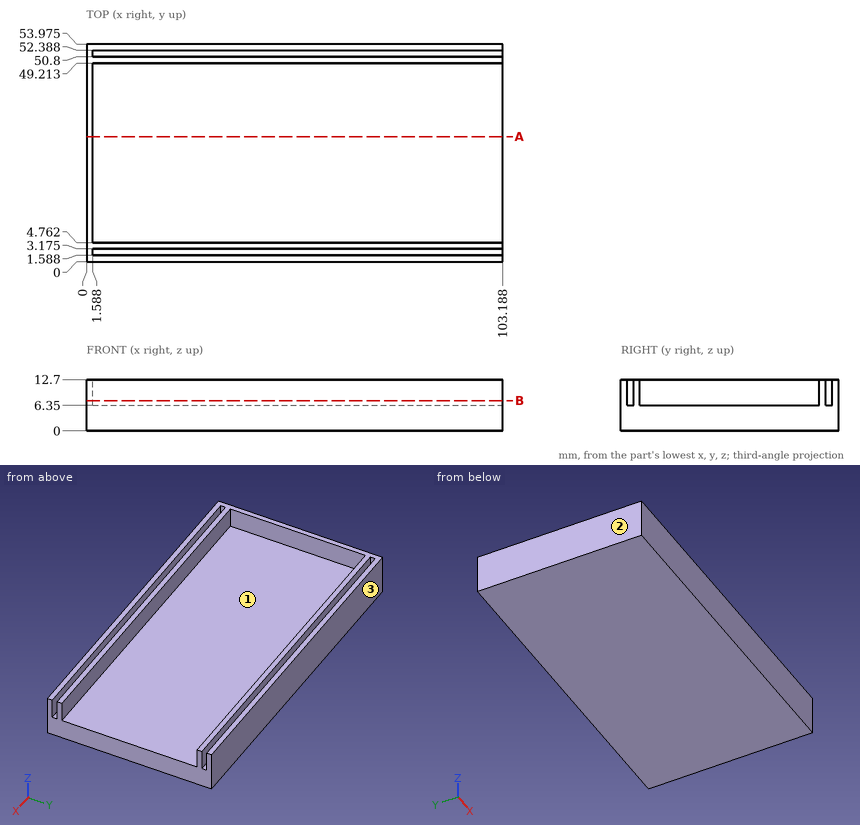
Here's the drawing with two shaded views (mm, measured from the low corner). I have some questions. Round coordinates to 2 decimals unless told otherwise and drop trailing zeros. Order: outer loops, then holes, each group sorted by start corner. A loop starts at its lowest first (then second) coordinate and runs counter-clockwise, first axis right, second up. Notation, with made-up numbers: (58.25, -5) -> (105.25, -5) arc R14 ccw to (105.25, 5) -> close; hole circle Ø7 at (53, -39). An arc over 180 degrees is marked (long way). Use a Markdown table: item, result. Add a question column.
(1) For pin 1 Ø12 at (x, y) = (19.5, 25.5) entering from +Z; pin 2 Ø1.9 at (y, z) = (26.5, 10) entering from +X, each with a flat end and sliding along its axis, tell me the tip position at first contact or that it passes through.
(2) Suppose I cut it at B-B, the plane z = 7.5. Please give me the cut outline in (x, y) (1 decimal).
(3) Suppose I cut it at A-A, the plane y = 31. Please give me the cut outline in (x, z).
(4) If we mould it in two halves opening along Y, with no side actions, what happens to the marked faces 1, 2 and 3? For each: released by +Y, released by -Y, zero draft, split by the parting line, or undercut.
(5) I need wall thicknesses on line 1 along Y through (x, z) = (83, 10) (1 decimal); line 2 along Z through (x, y) = (31.5, 26); line 3 along X through (y, z) = (22.5, 10.75). Which ranges of each line are inside material? Lowest first, please.
Verdict:
| question | item | result |
|---|---|---|
| 1 | pin 1 | z = 6.35 |
| 1 | pin 2 | x = 1.59 |
| 2 | outline | (0, 0) -> (103.2, 0) -> (103.2, 1.6) -> (1.6, 1.6) -> (1.6, 3.2) -> (103.2, 3.2) -> (103.2, 4.8) -> (1.6, 4.8) -> (1.6, 49.2) -> (103.2, 49.2) -> (103.2, 50.8) -> (1.6, 50.8) -> (1.6, 52.4) -> (103.2, 52.4) -> (103.2, 54) -> (0, 54) -> close |
| 3 | outline | (0, 0) -> (103.19, 0) -> (103.19, 6.35) -> (1.59, 6.35) -> (1.59, 12.7) -> (0, 12.7) -> close |
| 4 | face 1 | undercut |
| 4 | face 2 | zero draft |
| 4 | face 3 | released by +Y |
| 5 | line 1 | 0 to 1.6, 3.2 to 4.8, 49.2 to 50.8, 52.4 to 54 |
| 5 | line 2 | 0 to 6.35 |
| 5 | line 3 | 0 to 1.59 |
